from build123d import *

# Parameters (mm, degrees)
SKETCH1_R           = 22
SKETCH1_R_2         = 15
BOSS_EXTRUDE1_DEPTH = 3
SKETCH3_R           = 2.5
BOSS_EXTRUDE2_DEPTH = 24
SKETCH4_R           = 1.5
CUT_EXTRUDE1_DEPTH  = 6
SKETCH5_R           = 1.5
CUT_EXTRUDE2_DEPTH  = 6


with BuildPart() as part:
    # Sketch1 → Boss-Extrude1 (new body)
    with BuildSketch(Plane(origin=(0, 0, 0), x_dir=(1, 0, 0), z_dir=(0, 1, 0))):
        with Locations(Location((0, 0, 0), (0, 0, 270))):
            Circle(SKETCH1_R)
        with Locations(Location((0, 0, 0), (0, 0, 270))):
            Circle(SKETCH1_R_2, mode=Mode.SUBTRACT)
    extrude(amount=BOSS_EXTRUDE1_DEPTH)

    # Sketch3 → Boss-Extrude2 (add)
    with BuildSketch(Plane(origin=(0, 3, 0), x_dir=(1, 0, 0), z_dir=(0, 1, 0))):
        with Locations(Location((0, 18.5, 0), (0, 0, 270))):
            Circle(SKETCH3_R)
        with Locations(Location((18.5, 0, 0), (0, 0, 270))):
            Circle(SKETCH3_R)
        with Locations(Location((0, -18.5, 0), (0, 0, 270))):
            Circle(SKETCH3_R)
        with Locations(Location((-18.5, 0, 0), (0, 0, 270))):
            Circle(SKETCH3_R)
    extrude(amount=BOSS_EXTRUDE2_DEPTH)

    # Sketch4 → Cut-Extrude1 (cut)
    with BuildSketch(Plane(origin=(0, 27, 0), x_dir=(1, 0, 0), z_dir=(0, 1, 0))):
        with Locations(Location((-18.5, 0, 0), (0, 0, 270))):
            Circle(SKETCH4_R)
        with Locations(Location((0, 18.5, 0), (0, 0, 270))):
            Circle(SKETCH4_R)
        with Locations(Location((18.5, 0, 0), (0, 0, 270))):
            Circle(SKETCH4_R)
        with Locations(Location((0, -18.5, 0), (0, 0, 270))):
            Circle(SKETCH4_R)
    extrude(amount=-CUT_EXTRUDE1_DEPTH, mode=Mode.SUBTRACT)

    # Sketch5 → Cut-Extrude2 (cut)
    with BuildSketch(Plane(origin=(0, 3, 0), x_dir=(1, 0, 0), z_dir=(0, 1, 0))):
        with Locations(Location((13.081475452, 13.081475452, 0), (0, 0, 270))):
            Circle(SKETCH5_R)
        with Locations(Location((13.081475452, -13.081475452, 0), (0, 0, 270))):
            Circle(SKETCH5_R)
        with Locations(Location((-13.081475452, -13.081475452, 0), (0, 0, 270))):
            Circle(SKETCH5_R)
        with Locations(Location((-13.081475452, 13.081475452, 0), (0, 0, 270))):
            Circle(SKETCH5_R)
    extrude(amount=-CUT_EXTRUDE2_DEPTH, mode=Mode.SUBTRACT)


solid = part.part
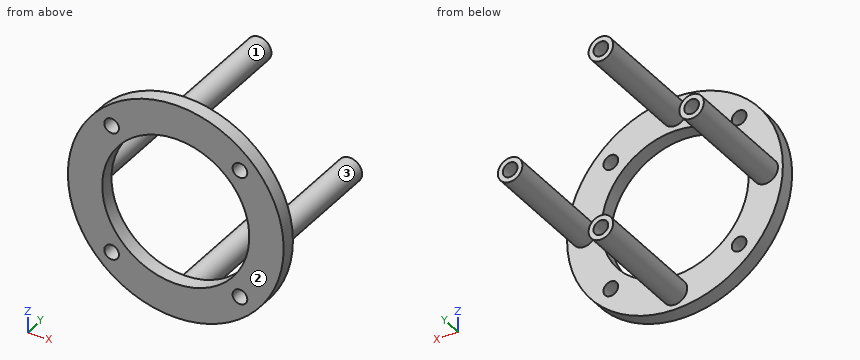
Check sheet for the modelled part. Datum: model origin and axes. Units: mm. Face numbers are marked on the shaded views. Round coordinates to 2 decimals unless told otherwise and drop trailing zeros. Loops run counter-clockwise (first coordinate to the right, second up) from the corner with the lowest first, then second, coordinate; pieces in that order, holes last.
1. Scan lines: probe 1 along X at (y, z) = (24.5, -18.5); probe 2 along X at (y, z) = (12, 2); probe 3 along Y at (x, z) = (-6, -20). Record each from-to range of solid material in increasing order.
2. Sectioned sample at D-D on y = 6.5. Record the boundary of the cut face in (x, z).
3. Sectioned sample at C-C on z = -11. Record the boundary of the cut face in (x, y), and give its area (3 significant figures).
4. Gauge pin test, flat ends, axial feed: pin 1 Ø5 at (x, z) = (13.08, 13.08) entering from +Y; pin 2 Ø0.9 at (x, z) = (0, -18.5) entering from +Y; pin 3 Ø1.5 at (y, z) = (16, 1) entering from -X. Record the tip position at first contact, or that the pin passes through.
5. Sectioned sample at B-B on x = 0. Record the boundary of the cut face in (y, z), and give its area (3 significant figures).
6. Mould release check, pull along X, two halves, no side actions. Record for the marked faces 1, 2 and 3: released by +X, released by -X, zero draft, split by the parting line, or undercut.
7. Sectioned sample at A-A on y = 23.75. Record the boundary of the cut face in (x, z).
Recorded:
1. probe 1: x = -2.5 to -1.5, 1.5 to 2.5
1. probe 2: x = -20 to -17, 17 to 20
1. probe 3: y = 0 to 3
2. outline: circle Ø5 at (-18.5, 0); circle Ø5 at (0, -18.5); circle Ø5 at (0, 18.5); circle Ø5 at (18.5, 0)
3. outline: (-19.05, 0) - (-10.2, 0) - (-10.2, 3) - (-19.05, 3) - close; (10.2, 0) - (19.05, 0) - (19.05, 3) - (10.2, 3) - close
3. area: 53.1 mm2
4. pin 1: stops at y = 3
4. pin 2: stops at y = 21
4. pin 3: stops at x = -20.99
5. outline: (0, -22) - (3, -22) - (3, -21) - (27, -21) - (27, -20) - (21, -20) - (21, -17) - (27, -17) - (27, -16) - (3, -16) - (3, -15) - (0, -15) - close; (0, 15) - (3, 15) - (3, 16) - (27, 16) - (27, 17) - (21, 17) - (21, 20) - (27, 20) - (27, 21) - (3, 21) - (3, 22) - (0, 22) - close
5. area: 246 mm2
6. face 1: split by the parting line
6. face 2: zero draft
6. face 3: undercut
7. outline: circle Ø5 at (-18.5, 0); circle Ø5 at (0, -18.5); circle Ø5 at (0, 18.5); circle Ø5 at (18.5, 0); hole circle Ø3 at (-18.5, 0); hole circle Ø3 at (0, -18.5); hole circle Ø3 at (0, 18.5); hole circle Ø3 at (18.5, 0)
